Design review of the part built by this model. Coordinates are the model's own, in mm. Face numbers are marked on the shaded views. Give positions to 0.01 mm unless a question says otherwise; leave off trailing zeros. Loops run counter-clockwise (first coordinate to the right, second up) from the corner with the lowest first, then second, coordinate; pieces in that order, holes last. Notation, with made-up numbers: (89.25, 1.5) -> (133.25, 1.5) arc R19 ccw to (133.25, 16.5) -> close; hole circle Ø9 at (12.25, -7). An arc over 180 degrees is marked (long way). Answer as CSV lines item,"result".
from build123d import *

# Parameters (mm, degrees)
BOSS_EXTRUDE2_DEPTH = 10
FILLET2_R           = 5
SKETCH3_W           = 46
SKETCH3_H           = 40
CUT_EXTRUDE1_DEPTH  = 4
SKETCH4_R           = 3
CUT_EXTRUDE2_DEPTH  = 6
CUT_EXTRUDE3_START  = -2
SKETCH5_R           = 2
CUT_EXTRUDE3_DEPTH  = 8


with BuildPart() as part:
    # Sketch1 → Boss-Extrude2 (new body)
    with BuildSketch(Plane(origin=(0, 0, 0), x_dir=(1, 0, 0), z_dir=(0, 1, 0))):
        with BuildLine():
            Line((-112.915113285, 9.992897111), (-102.291556109, -20.007102889))
            ThreePointArc((-102.291556109, -20.007102889), (-96.809111593, -27.249623327), (-88.151933742, -30))
            Line((-88.151933742, -30), (88.151933742, -30))
            ThreePointArc((88.151933742, -30), (96.809111593, -27.249623327), (102.291556109, -20.007102889))
            Line((102.291556109, -20.007102889), (112.915113285, 9.992897111))
            ThreePointArc((112.915113285, 9.992897111), (111.025114246, 23.657177851), (98.775490918, 30))
            Line((98.775490918, 30), (-98.775490918, 30))
            ThreePointArc((-98.775490918, 30), (-111.025114246, 23.657177851), (-112.915113285, 9.992897111))
        make_face()
    extrude(amount=BOSS_EXTRUDE2_DEPTH)

    # Fillet2
    fillet2_edges = [part.edges().sort_by_distance(p)[0] for p in [
        (111.025114246, 10, -23.657177851),
        (0, 0, -30),
        (-111.025114246, 0, -23.657177851),
        (107.603334697, 10, 5.007102889),
        (96.809111593, 10, 27.249623327),
        (0, 10, 30),
        (-96.809111593, 10, 27.249623327),
        (-107.603334697, 10, 5.007102889),
        (0, 10, -30),
        (-107.603334697, 0, 5.007102889),
        (0, 0, 30),
        (107.603334697, 0, 5.007102889),
    ]]
    fillet(fillet2_edges, radius=FILLET2_R - 0.0001)  # a hair under: the kernel refuses the full size

    # Sketch3 → Cut-Extrude1 (cut)
    with BuildSketch(Plane(origin=(0, 10, 0), x_dir=(1, 0, 0), z_dir=(0, 1, 0))):
        Rectangle(SKETCH3_W, SKETCH3_H)
    extrude(amount=-CUT_EXTRUDE1_DEPTH, mode=Mode.SUBTRACT)

    # Sketch4 → Cut-Extrude2 (cut)
    with BuildSketch(Plane(origin=(0, 6, 0), x_dir=(1, 0, 0), z_dir=(0, 1, 0))):
        with Locations(Location((12, 0, 0), (0, 0, 270))):
            Circle(SKETCH4_R)
        with Locations(Location((-12, 0, 0), (0, 0, 90))):
            Circle(SKETCH4_R)
    extrude(amount=-CUT_EXTRUDE2_DEPTH, mode=Mode.SUBTRACT)

    # Sketch5 → Cut-Extrude3 (cut)
    with BuildSketch(Plane(origin=(0, 10, 0), x_dir=(1, 0, 0), z_dir=(0, 1, 0)).offset(CUT_EXTRUDE3_START)):
        with Locations(Location((-70, 8, 0), (0, 0, 270))):
            Circle(SKETCH5_R)
        with Locations(Location((-70, -8, 0), (0, 0, 90))):
            Circle(SKETCH5_R)
        with Locations(Location((70, -8, 0), (0, 0, 270))):
            Circle(SKETCH5_R)
        with Locations(Location((70, 8, 0), (0, 0, 90))):
            Circle(SKETCH5_R)
    extrude(amount=-CUT_EXTRUDE3_DEPTH, mode=Mode.SUBTRACT)


solid = part.part
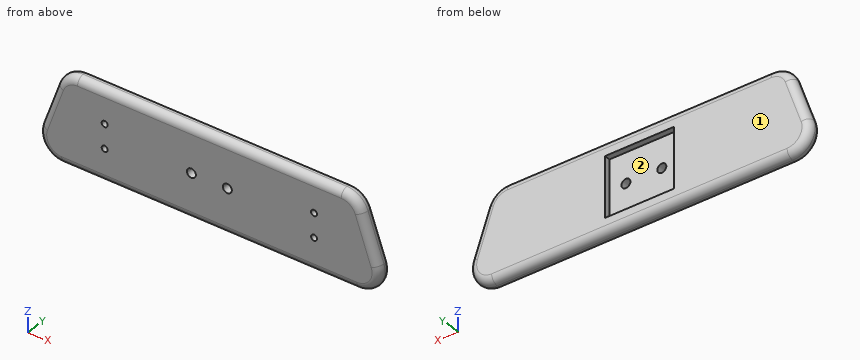
Q1. The part is to be moulded in two halves that separate along Z. For the marked faces 1 and 2, say which applies: pulls with the +Z half, pulls with the -Z half, needs draft (parallel to the pull), parting line crosses it, or undercut.
Filled sheet:
face 1,"needs draft"
face 2,"undercut"
Q2. We need section D-D, the plane z = 0. State how many separate pieces and enclosed holes the cut face has, and give its area (3 significant figures).
Filled sheet:
separate pieces,"3"
enclosed holes,"0"
area,"1,910 mm^2"
Q3. We need section C-C, the plane y = 2.25. State the section outline as (x, z) points.
Filled sheet:
outline,"(-112.14, -10.27) arc R14.18 ccw to (-98.78, -29.18) -> (98.78, -29.18) arc R14.18 ccw to (112.14, -10.27) -> (101.51, 19.73) arc R14.18 ccw to (88.15, 29.18) -> (-88.15, 29.18) arc R14.18 ccw to (-101.51, 19.73) -> close; hole circle Ø4 at (-70, -8); hole circle Ø4 at (-70, 8); hole circle Ø6 at (-12, 0); hole circle Ø6 at (12, 0); hole circle Ø4 at (70, -8); hole circle Ø4 at (70, 8)"
Q4. To check wall thickness, follow probe 1 along X at (y, z) = (1, 0.5); probe 2 along X at (y, z) = (4.25, 8); probe 3 along X at (y, z) = (9, -7). State the ranges of each line that lie inside material, in increasing order. Write a range as from..to.
Filled sheet:
probe 1,"x = -107.08..-14.96, -9.04..9.04, 14.96..107.08"
probe 2,"x = -106.48..-72, -68..68, 72..106.48"
probe 3,"x = -109.73..-23, 23..109.73"
Q5. Clearance check with flat-ended pins moving along their axes: pin 1 Ø5 at (y, z) = (3.5, 6.5) entering from -X; pin 2 Ø2 at (y, z) = (7.5, -3.5) entering from +X; pin 3 Ø3 at (x, z) = (-70, 8) entering from -Y. State where each tip first meets the part, or that it passes through.
Filled sheet:
pin 1,"stops at x = -107.86"
pin 2,"stops at x = 110.51"
pin 3,"stops at y = 8"
